Part model, mm, in its own coordinate system. A direction names the side the tool comes from. Round coordinates to 2 decimals unless told otherwise and drop trailing zeros. Loops run counter-clockwise (first coordinate to the right, second up) from the corner with the lowest first, then second, coordinate; pieces in that order, holes last. Notation, with made-up numbers: (43, 22) - (48, 22) arc R12 cw to (48, 27) - close; hole circle Ø2 at (11.25, 34.5). An arc over 180 degrees is marked (long way). Put each result on its own line as item: value.
from build123d import *

# Parameters (mm, degrees)
SKETCH_3_R        = 4.5
EXTRUDE_1_DEPTH   = 9
SKETCH_4_W        = 1
SKETCH_4_H        = 0.3
SKETCH_6_R        = 0.7
EXTRUDE_2_DEPTH   = 6
EXTRUDE_2_2_DEPTH = 6
SKETCH_7_R        = 0.7


with BuildPart() as part:
    # Sketch 3 → Extrude 1 (new body)
    with BuildSketch(Plane(origin=(6.5, 0, 0), x_dir=(0, 0, -1), z_dir=(1, 0, 0))):
        with Locations((-1.525, -0.033649265)):
            Circle(SKETCH_3_R)
    extrude(amount=EXTRUDE_1_DEPTH)

    # Sketch 4 → Cut-Revolve 1 (revolve, cut)
    with BuildSketch(Plane(origin=(0, 0, 0), x_dir=(1, 0, 0), z_dir=(0, 1, 0)), mode=Mode.PRIVATE) as cut_revolve_1_sk:
        with Locations((7.7, 2.925)):
            Rectangle(SKETCH_4_W, SKETCH_4_H)
    revolve(cut_revolve_1_sk.sketch.rotate(Axis((0, 0, 1.525), (1, 0, 0)), 180), axis=Axis((0, 0, 1.525), (1, 0, 0)), mode=Mode.SUBTRACT)



with BuildPart() as body_2:
    # Sketch 6 → Extrude 2 (new body)
    with BuildSketch(Plane.XY):
        Circle(SKETCH_6_R)
    extrude(amount=-EXTRUDE_2_DEPTH)


with BuildPart() as body_3:
    # Sketch 6 → Extrude 2 2 (new body)
    with BuildSketch(Plane.XY):
        with Locations(Location((22, 0, 0), (0, 0, 180))):
            Circle(SKETCH_6_R)
    extrude(amount=-EXTRUDE_2_2_DEPTH)


with BuildPart() as part_1:
    add(part.part)

    add(body_2.part)  # Sweep 1 merges body 2

    add(body_3.part)  # Sweep 1 merges body 3
    # Sweep 1: sweep along a path in Sketch 5
    with BuildLine(Plane(origin=(0, 0, 0), x_dir=(1, 0, 0), z_dir=(0, 1, 0))) as sweep_1_path:
        Line((0, 0), (0, -0.525))
        ThreePointArc((0, -0.525), (0.292893219, -1.232106781), (1, -1.525))
        Line((1, -1.525), (6.8, -1.525))
        Line((6.8, -1.525), (21, -1.525))
        ThreePointArc((21, -1.525), (21.707106781, -1.232106781), (22, -0.525))
        Line((22, -0.525), (22, 0))
    # Sketch 7 → Sweep 1 (sweep)
    with BuildSketch(Plane.XY):
        Circle(SKETCH_7_R)
    sweep(path=sweep_1_path.line)


solid = part_1.part
1. Probe line 1 along X through (y, z) = (2.5, -0.5); line 2 along Y through (x, z) = (15.25, 3); line 3 along Y through (x, z) = (5.75, 1). List the from-to ranges inside material, lowest first. Write a range as [from, to].
A:
line 1: x = [6.5, 15.5]
line 2: y = [-4.29, 4.22]
line 3: y = [-0.46, 0.46]
2. Pin check, flat tips, straight feed: P1, Ø2.5, axis at y = 0.5, z = -0.5, coming from the -X side; P2, Ø1.5, axis at x = 8.5, z = 3.5, coming from the -Y side; P3, Ø4, axis at y = -2, z = 4, coming from the +X side; P4, Ø1.5, axis at x = 11.5, y = -2, coming from the +Z side. Stop position of each tip, or through.
A:
P1: stops at x = -0.7
P2: stops at y = -4.36
P3: stops at x = 15.5
P4: stops at z = 5.86
3. Tool access for faces 3 (the cylindrical face through (-0.7, 0, -2.7)), 4 (the cylindrical face through (18.288, 0.031, 2.224)), 5 (the flat face through (0, 0, -6)): list every direction of +Z, -Z, +X, -X, +Y, -Y with a clear straight run to the whole face (end or side of a thin tool).
A:
face 3: -Z
face 4: none
face 5: -Z, +X, -X, +Y, -Y
4. Band-saw the part on A-A (z = -4.5). List the corners of the cut face in (x, y).
A:
outline: circle Ø1.4 at (0, 0); circle Ø1.4 at (22, 0)
5. Band-saw the part on D-D (x = 4.25). List the corners of the cut face in (y, z) (3 decimals), plus the area to 3 significant figures.
A:
outline: circle Ø1.4 at (0, 1.525)
area: 1.54 mm²
6. Band-saw the part on B-B (y = 1). List the corners of the cut face in (x, z), plus the area to 3 significant figures.
A:
outline: (6.5, -2.85) - (7.2, -2.85) - (7.2, -2.66) - (8.2, -2.66) - (8.2, -2.85) - (15.5, -2.85) - (15.5, 5.9) - (8.2, 5.9) - (8.2, 5.71) - (7.2, 5.71) - (7.2, 5.9) - (6.5, 5.9) - close
area: 78.4 mm²
7. Band-saw the part on C-C (z = 4.25). List the corners of the cut face in (x, y), plus the area to 3 significant figures.
A:
outline: (6.5, -3.61) - (7.2, -3.61) - (7.2, -3.33) - (8.2, -3.33) - (8.2, -3.61) - (15.5, -3.61) - (15.5, 3.55) - (8.2, 3.55) - (8.2, 3.33) - (7.2, 3.33) - (7.2, 3.55) - (6.5, 3.55) - close
area: 64.0 mm²
8. Two-plate mould, pull along X, no slides. Class faces 1 (the flat face through (22, 0, -6)), 2 (the cylindrical face through (21.332, 0.21, -2.783)): pulls with the +X half, pulls with the -X half, needs draft (parallel to the pull), parting line crosses it, or undercut.
A:
face 1: needs draft
face 2: undercut
